from build123d import *

# Parameters (mm, degrees)
SKETCH1_W           = 20
SKETCH1_H           = 30
SKETCH1_R           = 4.7625
BOSS_EXTRUDE1_DEPTH = 10
SKETCH2_W           = 20
SKETCH2_H           = 10
BOSS_EXTRUDE2_DEPTH = 19
SKETCH3_R           = 1.5
CUT_EXTRUDE1_DEPTH  = 51


with BuildPart() as part:
    # Sketch1 → Boss-Extrude1 (new body)
    with BuildSketch(Plane.XY):
        with Locations((10, 15)):
            Rectangle(SKETCH1_W, SKETCH1_H)
        with Locations((10, 15)):
            Circle(SKETCH1_R, mode=Mode.SUBTRACT)
    extrude(amount=BOSS_EXTRUDE1_DEPTH)

    # Sketch2 → Boss-Extrude2 (add)
    with BuildSketch(Plane.XY):
        with Locations((10, -5)):
            Rectangle(SKETCH2_W, SKETCH2_H)
        with Locations((10, 35)):
            Rectangle(SKETCH2_W, SKETCH2_H)
    extrude(amount=BOSS_EXTRUDE2_DEPTH)

    # Sketch3 → Cut-Extrude1 (cut, through all)
    with BuildSketch(Plane(origin=(0, 40, 0), x_dir=(1, 0, 0), z_dir=(0, 1, 0))):
        with Locations((10, -14.5)):
            Circle(SKETCH3_R)
    extrude(amount=-CUT_EXTRUDE1_DEPTH, mode=Mode.SUBTRACT)


solid = part.part
CAD build for the part. Positions are in the model's coordinates, mm. A direction names the side the tool comes from. Give positions to 0.01 mm unless a question says otherwise; leave off trailing zeros. Write each loop counter-clockwise with the first axis right and the second up, starting at its lowest first coordinate (ties: lowest second). Pieces come first, ordered by that corner, then holes. Notation, with made-up numbers: (44, -31) - (102, -31) arc R14 ccw to (102, -21) - close; hole circle Ø8 at (46.5, 70.5). An arc over 180 degrees is marked (long way). Put each result on its own line as item: value.
(1) Saw through at C-C (y = 15). List the corners of the cut face in (x, z).
Working result:
outline: (0, 0) - (5.24, 0) - (5.24, 10) - (0, 10) - close; (14.76, 0) - (20, 0) - (20, 10) - (14.76, 10) - close
(2) Saw through at B-B (x = 10). List the corners of the cut face in (y, z), then the cut area to 3 significant figures.
Working result:
outline: (-10, 0) - (10.24, 0) - (10.24, 10) - (0, 10) - (0, 13) - (-10, 13) - close; (-10, 16) - (0, 16) - (0, 19) - (-10, 19) - close; (19.76, 0) - (40, 0) - (40, 13) - (30, 13) - (30, 10) - (19.76, 10) - close; (30, 16) - (40, 16) - (40, 19) - (30, 19) - close
area: 525 mm^2
(3) Drop flat-ended pins along their axis: pin 1 Ø5 at (x, y) = (16, 17) entering from +Z; pin 2 Ø8.5 at (x, y) = (10, 15) entering from +Z (3 decimals). Give the stop position or say it passes through.
Working result:
pin 1: z = 10
pin 2: through
(4) Saw through at D-D (x = 15.25). List the corners of the cut face in (y, z).
Working result:
outline: (-10, 0) - (40, 0) - (40, 19) - (30, 19) - (30, 10) - (0, 10) - (0, 19) - (-10, 19) - close
(5) Tool access for faces 4 (the flat face through (0, 15, 7)), 5 (the flat face through (10, 0, 12)): list every direction of +Z, -Z, +X, -X, +Y, -Y with a clear straight run to the whole face (end or side of a thin tool).
Working result:
face 4: +Z, -Z, -X, +Y, -Y
face 5: +Z, +X, -X
(6) Wall check: L1, parallel to Y at x = 5, z = 11; L2, parallel to Y at x = 10, z = 6; L3, parallel to X at y = 37.5, z = 14.5. Give the ranges that are in metal, low to high.
Working result:
L1: -10 to 0, 30 to 40
L2: -10 to 10.24, 19.76 to 40
L3: 0 to 8.5, 11.5 to 20
(7) Pull direction Z, two halves, no side cores. Call faces 1 (the cylindrical face through (8.5, 35.07, 14.43)), 2 (the flat face through (10, 21, 0)), 3 (the cylindrical face through (12.198, 10.775, 4.93)): released by +Z, released by -Z, zero draft, split by the parting line, or undercut.
Working result:
face 1: undercut
face 2: released by -Z
face 3: zero draft
(8) Saw through at A-A (z = 14.5). List the corners of the cut face in (x, y), then the cut area to 3 significant figures.
Working result:
outline: (0, -10) - (8.5, -10) - (8.5, 0) - (0, 0) - close; (0, 30) - (8.5, 30) - (8.5, 40) - (0, 40) - close; (11.5, -10) - (20, -10) - (20, 0) - (11.5, 0) - close; (11.5, 30) - (20, 30) - (20, 40) - (11.5, 40) - close
area: 340 mm^2
